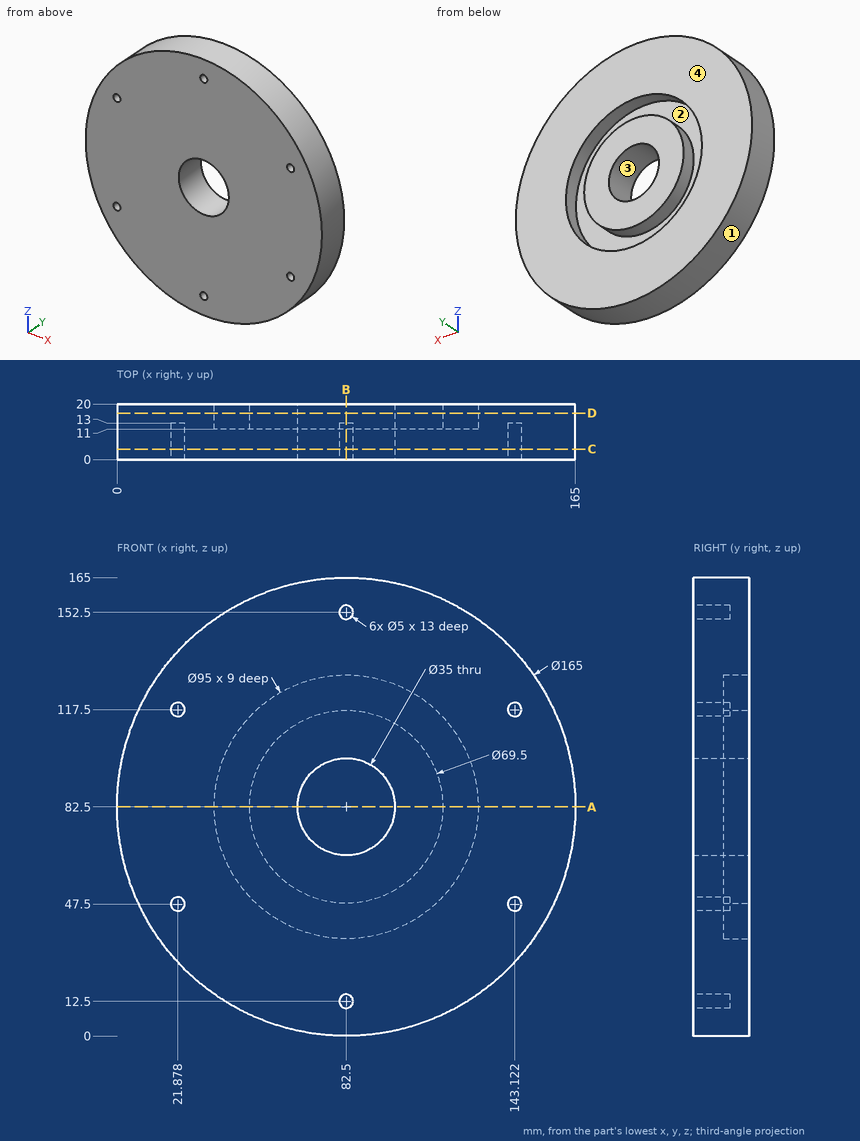
Answer from the drawing. Dimensions are ordinates in mm from the lowest x, y and z of the part. Coordinates: 2 decimals unless noted, no trailing zeros. Order: outer loops, then holes, each group sorted by start corner. A loop starts at its lowest first (then second) coordinate and runs counter-clockwise, first axis right, second up. Notation, with made-up numbers: M -2,33 L 51,33 A21 ccw 51,44 Z; hole C 27,45.5 d9. An arc over 180 degrees is marked long. Put each result on its own line as item: value. Start each with the question number.
Item 1: Section A-A, the plane z = 82.5 is taken. Determine the outline of the cut face in (x, y), plus the area to 3 significant figures.
Item 2: Section C-C, the plane y = 3.75 is taken. Determine the outline of the cut face in (x, z), plus the area to 3 significant figures.
Item 3: Consider probe 1 along Z at (x, y) = (82.5, 2.75); probe 2 along X at (y, z) = (16.75, 82.5); probe 3 along X at (y, z) = (7.25, 82.5). Determine where each line is inside the solid, lowest interval first. Write a range as [from, to].
Item 4: The mould has two halves that part along Z. Classify the marked faces 1, 2, 3 and 4: +Z half, -Z half, draft (parallel to the pull), parting line (faces both ways), or undercut.
Item 5: Section D-D, the plane y = 16.75 is taken. Determine the outline of the cut face in (x, z), plus the area to 3 significant figures.
Item 6: Section B-B, the plane x = 82.5 is taken. Determine the outline of the cut face in (y, z).
Item 7: Given pin 1 Ø1.5 at (x, z) = (81.5, 151.5) entering from -Y; pin 2 Ø3 at (x, y) = (43, 10.5) entering from +Z; pin 3 Ø2 at (y, z) = (11, 97) entering from +X, each flat-ended and moving along its own axis, determine where each tip first touches the part or whether it passes through.
Computed:
1. outline: M 0,0 L 65,0 L 65,20 L 47.75,20 L 47.75,11 L 35,11 L 35,20 L 0,20 Z; M 100,0 L 165,0 L 165,20 L 130,20 L 130,11 L 117.25,11 L 117.25,20 L 100,20 Z
1. area: 2,370 mm2
2. outline: C 82.5,82.5 d165; hole C 21.88,47.5 d5; hole C 21.88,117.5 d5; hole C 82.5,82.5 d35; hole C 82.5,12.5 d5; hole C 82.5,152.5 d5; hole C 143.12,47.5 d5; hole C 143.12,117.5 d5
2. area: 20,300 mm2
3. probe 1: z = [0, 10], [15, 65], [100, 150], [155, 165]
3. probe 2: x = [0, 35], [47.75, 65], [100, 117.25], [130, 165]
3. probe 3: x = [0, 65], [100, 165]
4. face 1: parting line
4. face 2: undercut
4. face 3: undercut
4. face 4: draft
5. outline: C 82.5,82.5 d165; C 82.5,82.5 d69.5; hole C 82.5,82.5 d95; hole C 82.5,82.5 d35
5. area: 17,100 mm2
6. outline: M 0,0 L 20,0 L 20,35 L 11,35 L 11,47.75 L 20,47.75 L 20,65 L 0,65 L 0,15 L 13,15 L 13,10 L 0,10 Z; M 0,100 L 20,100 L 20,117.25 L 11,117.25 L 11,130 L 20,130 L 20,165 L 0,165 L 0,155 L 13,155 L 13,150 L 0,150 Z
7. pin 1: stops at y = 13
7. pin 2: stops at z = 155.73
7. pin 3: stops at x = 163.89
